Can you work these out from the model? Positions are in its coordinate system, mm. Face numbers are marked on the shaded views. A direction names the side the tool comes from. Round coordinates to 2 decimals unless told otherwise and drop trailing zeros. Write item = value, one per line.
from build123d import *

# Parameters (mm, degrees)
F1_R     = 25.4
F2_DEPTH = 25.4
F3_R     = 25.39999
F4_R     = 16.1798
F5_DEPTH = 2.54


# Not quite as in the source:
# - a variable given as a bare number and used for a length is read in inches; the dataset says mm whatever the document's units were
# - a fillet or chamfer is up to 0.001 mm smaller than in the source, because OpenCascade refuses the exact size


with BuildPart() as f2:
    # F1 (on Top) → F2 (new body)
    with BuildSketch(Plane.XY):
        Circle(F1_R)
    extrude(amount=F2_DEPTH)

    # F3 (radius 25.4 in the source; OpenCascade refuses exactly that, so slightly less here)
    f3_edges = [f2.edges().sort_by_distance(p)[0] for p in [
        (-25.4, 0, 25.4),
    ]]
    fillet(f3_edges, radius=F3_R)

    # F4 (on face) → F5 (join)
    with BuildSketch(Plane(origin=(0, 0, 0), x_dir=(1, 0, 0), z_dir=(0, 0, -1))):
        Circle(F4_R)
    extrude(amount=F5_DEPTH)


solid = f2.part
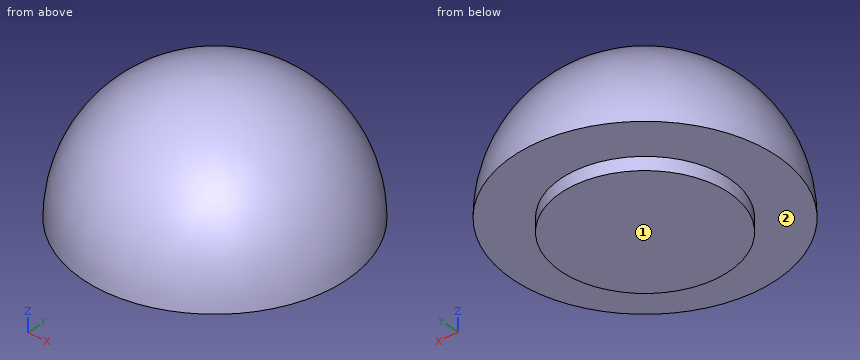
(1) If I drill on line 1 (X direction, y = -3, z = 22.75); line 2 (Z direction, x = 4, y = -4.5), over which ranges is the centre line in solid material (lowest first)? Write a range as from..to.
Computed:
line_1 = -10.89..10.89
line_2 = -2.54..24.68
(2) Will these pins go through, and if not, where does the flat tip stop? P1, Ø6, axis at x = -8, y = 0, coming from the +Z side; P2, Ø8, axis at x = -19.5, y = -13, coming from the -Z side; P3, Ø1.5, axis at y = -16.5, z = 9, coming from the -X side.
Computed:
P1 = 24.9
P2 = 0
P3 = -17.88
(3) On a 3-axis mill with a long thin cutter (end or side, diameter ignored), from which of +Z, -Z, +X, -X, +Y, -Y can I reach the whole of each face in a straight line? I mean the marked faces 1 and 2. Say none if no direction works.
Computed:
face_1 = -Z, +X, -X, +Y, -Y
face_2 = -Z
